```python
from build123d import *

# Parameters (mm, degrees)
SKETCH_W     = 57
SKETCH_H     = 57
PAD_DEPTH    = 5
FILLET_R     = 3
SKETCH001_R  = 28
PAD001_DEPTH = 48
SKETCH002_R  = 3.175
PAD002_DEPTH = 10
SKETCH003_R  = 19
PAD003_DEPTH = 1
SKETCH004_R  = 3
POCKET_DEPTH = 53.001


with BuildPart() as part:
    # Sketch → Pad (new body)
    with BuildSketch(Plane.XZ):
        with Locations((28.5, 28.5)):
            Rectangle(SKETCH_W, SKETCH_H)
    extrude(amount=-PAD_DEPTH)

    # Fillet
    fillet_edges = [part.edges().sort_by_distance(p)[0] for p in [
        (0, 2.5, 0),
        (57, 2.5, 0),
        (57, 2.5, 57),
        (0, 2.5, 57),
    ]]
    fillet(fillet_edges, radius=FILLET_R)

    # Sketch001 → Pad001 (new body)
    with BuildSketch(Plane.XZ):
        with Locations((28.5, 28.5)):
            Circle(SKETCH001_R)
    extrude(amount=PAD001_DEPTH)

    # Sketch002 → Pad002 (new body)
    with BuildSketch(Plane(origin=(0, 5, 0), x_dir=(-1, 0, 0), z_dir=(0, 1, 0))):
        with Locations((-28.5, 28.5)):
            Circle(SKETCH002_R)
    extrude(amount=PAD002_DEPTH)

    # Sketch003 → Pad003 (new body)
    with BuildSketch(Plane(origin=(0, 5, 0), x_dir=(-1, 0, 0), z_dir=(0, 1, 0))):
        with Locations((-28.5, 28.5)):
            Circle(SKETCH003_R)
    extrude(amount=PAD003_DEPTH)

    # Sketch004 → Pocket (cut, through all)
    with BuildSketch(Plane(origin=(0, 5, 0), x_dir=(-1, 0, 0), z_dir=(0, 1, 0))):
        with Locations((-52.5, 52.5)):
            Circle(SKETCH004_R)
        with Locations((-4.5, 52.5)):
            Circle(SKETCH004_R)
        with Locations((-52.5, 4.5)):
            Circle(SKETCH004_R)
        with Locations((-4.5, 4.5)):
            Circle(SKETCH004_R)
    extrude(amount=-POCKET_DEPTH, mode=Mode.SUBTRACT)


solid = part.part
```
Source: CAD feature listing. Evaluate the final solid. Frame: model axes, mm. A direction names the side the tool comes from. Give positions to 0.01 mm unless a question says otherwise; leave off trailing zeros. Loops run counter-clockwise (first coordinate to the right, second up) from the corner with the lowest first, then second, coordinate; pieces in that order, holes last. Notation, with made-up numbers: M 15.5,8.5 L 69.5,8.5 A22 ccw 69.5,27.5 Z; hole C 72,38.25 d8. An arc over 180 degrees is marked long. Put each result on its own line as item: value.
Q1. Pin query (flat end, axial travel): P1, Ø7, axis at x = 4.5, z = 52.5, coming from the -Y side; P2, Ø4, axis at y = -13.5, z = 39, coming from the +X side; P3, Ø3, axis at x = 44, y = -10, coming from the -Z side; P4, Ø3.5, axis at x = 52.5, z = 4.5, coming from the +Y side. Return the tip coordinate at first contact, or that it passes through.
Response values:
P1: stops at y = 0
P2: stops at x = 55.18
P3: stops at z = 4.25
P4: passes through
Q2. Section C-C (x = 4.5). Return the cut outline in (y, z), and give its area (3 significant figures).
Response values:
outline: M -48,14.08 L 0,14.08 L 0,7.5 L 5,7.5 L 5,49.5 L 0,49.5 L 0,42.92 L -48,42.92 Z; M 0,0 L 5,0 L 5,1.5 L 0,1.5 Z; M 0,55.5 L 5,55.5 L 5,57 L 0,57 Z
area: 1,610 mm²
Q3. Reachability of faces 1 (the cylindrical face through (41.42, -23.66, 3.66)), 2 (the flat face through (9, 5, 29)), 3 (the flat face through (28, 2, 0)) from +Z, -Z, +X, -X, +Y, -Y: full face, straight path, thin tool, end or side. Return the list, or none.
Response values:
face 1: -Y
face 2: +Y
face 3: -Z, +X, -X, +Y, -Y
Q4. Section A-A (x = 28.5). Return the cut outline in (y, z) (3 decimals), and give its area (3 significant figures).
Response values:
outline: M -48,0.5 L 0,0.5 L 0,0 L 5,0 L 5,9.5 L 6,9.5 L 6,25.325 L 15,25.325 L 15,31.675 L 6,31.675 L 6,47.5 L 5,47.5 L 5,57 L 0,57 L 0,56.5 L -48,56.5 Z
area: 3,070 mm²
Q5. Section D-D (z = 28.5). Return the cut outline in (x, y) (3 decimals).
Response values:
outline: M 0,0 L 0.5,0 L 0.5,-48 L 56.5,-48 L 56.5,0 L 57,0 L 57,5 L 47.5,5 L 47.5,6 L 31.675,6 L 31.675,15 L 25.325,15 L 25.325,6 L 9.5,6 L 9.5,5 L 0,5 Z
Q6. Line query: probe 1 along Z at (x, y) = (52.5, 3.65); probe 2 along X at (y, z) = (3, 52); probe 3 along Y at (x, z) = (19.5, 28.5). Output: solid intervals per line, ascending. Write a range as [from, to].
Response values:
probe 1: z = [0, 1.5], [7.5, 49.5], [55.5, 57]
probe 2: x = [0, 1.54], [7.46, 49.54], [55.46, 57]
probe 3: y = [-48, 6]
Q7. Mould query, pull axis X, two halves, no side actions, for faces 4 (the cylindrical face through (55.5, 2.5, 4.6)), 5 (the flat face through (29, 15, 29)), 6 (the cylindrical face through (29.19, 10.44, 25.4)), 7 (the flat face through (57, 2, 28)). Classes: released by +X, released by -X, zero draft, split by the parting line, or undercut.
Response values:
face 4: undercut
face 5: zero draft
face 6: split by the parting line
face 7: released by +X
Q8. Section B-B (z = 6). Return the cut outline in (x, y), and give its area (3 significant figures).
Response values:
outline: M 0,0 L 1.9,0 L 1.9,5 L 0,5 Z; M 7.1,0 L 11.83,0 L 11.83,-48 L 45.17,-48 L 45.17,0 L 49.9,0 L 49.9,5 L 7.1,5 Z; M 55.1,0 L 57,0 L 57,5 L 55.1,5 Z
area: 1,830 mm²
